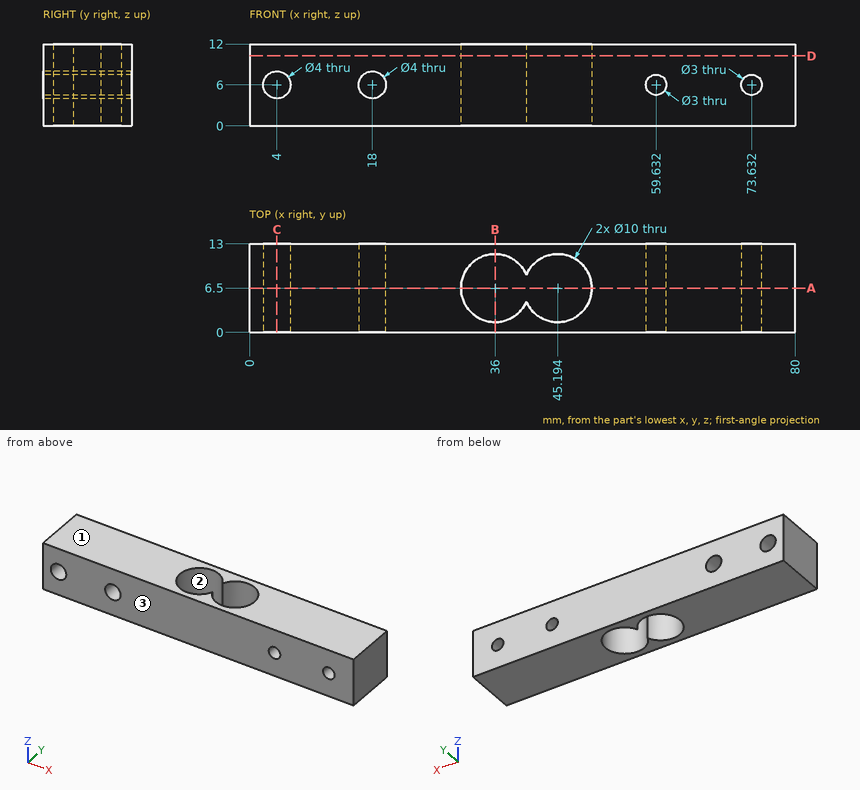
Job drawing, mm, ordinate dimensions from the low corner. One solid piece. Round coordinates to 2 decimals unless told otherwise and drop trailing zeros. Loops run counter-clockwise (first coordinate to the right, second up) from the corner with the lowest first, then second, coordinate; pieces in that order, holes last.
(1) Drop a flat-ended pin along its axis: pin 1 (5 mm diameter, centred on x = 45.5, y = 5, fed in from +Z). Give the stop position or say it passes through.
(2) Cut at B-B (x = 36). Give the cut face in (y, z), plus the area to 3 significant figures.
(3) Two-plate mould, pull along Y, no slides. Class the marked faces 1, 2 and 3: +Y half, -Y half, draft (parallel to the pull), parting line (faces both ways), or undercut.
(4) Cut at C-C (x = 4). Give the cut face in (y, z), plus the area to 3 significant figures.
(5) Wall check: line 1 along Y through (x, z) = (45, 9); line 2 along X through (y, z) = (5, 7.75) (1 decimal); line 3 along Z through (x, y) = (18, 9). Give the ranges that are in metal, low to high.
(6) Cut at A-A (y = 6.5). Give the cut face in (x, z).
(7) Cut at D-D (z = 10.25). Give the cut face in (x, y).
Findings below:
1. pin 1: passes through
2. outline: (0, 0) - (1.5, 0) - (1.5, 12) - (0, 12) - close; (11.5, 0) - (13, 0) - (13, 12) - (11.5, 12) - close
2. area: 36.0 mm2
3. face 1: draft
3. face 2: undercut
3. face 3: -Y half
4. outline: (0, 0) - (13, 0) - (13, 4) - (0, 4) - close; (0, 8) - (13, 8) - (13, 12) - (0, 12) - close
4. area: 104 mm2
5. line 1: y = 0 to 1.5, 11.5 to 13
5. line 2: x = 0 to 3, 5 to 17, 19 to 31.2, 50 to 80
5. line 3: z = 0 to 4, 8 to 12
6. outline: (0, 0) - (31, 0) - (31, 12) - (0, 12) - close; (50.19, 0) - (80, 0) - (80, 12) - (50.19, 12) - close; hole circle Ø4 at (4, 6); hole circle Ø4 at (18, 6); hole circle Ø3 at (59.63, 6); hole circle Ø3 at (73.63, 6)
7. outline: (0, 0) - (80, 0) - (80, 13) - (0, 13) - close; hole (40.6, 4.53) arc R5 ccw (long way) to (40.6, 8.47) arc R5 ccw (long way) to start
